Build history of the part. All positions in model axes, mm. A direction names the side the tool comes from. Round coordinates to 2 decimals unless told otherwise and drop trailing zeros. Loops run counter-clockwise (first coordinate to the right, second up) from the corner with the lowest first, then second, coordinate; pieces in that order, holes last. Notation, with made-up numbers: M 53,64.25 L 100,64.25 A20 cw 100,81.25 Z; hole C 8,71.25 d10. An arc over 180 degrees is marked long. Use one line per item in the form item = value. Start each with the question number.
Autodesk Inventor part; units mm, degrees
ref_plane "YZ Plane" through (0, 0, 0) normal (1, 0, 0) x (0, 1, 0)
ref_plane "XZ Plane" through (0, 0, 0) normal (0, 1, 0) x (-1, 0, 0)
ref_plane "XY Plane" through (0, 0, 0) normal (0, 0, 1) x (1, 0, 0)
sketch "Sketch1" plane through (0, 0, 0) normal (0, 0, 1) x (1, 0, 0)
  circle A0 centre (0, 0) radius 7.5
  line L0 (-10, 10) -> (10, 10)
  line L1 (10, 10) -> (10, -10)
  line L2 (10, -10) -> (-10, -10)
  line L3 (-10, -10) -> (-10, 10)
  line L4 (-10, -10) -> (-14, -10)
  line L5 (-14, -10) -> (-14, 10)
  line L6 (-14, 10) -> (-10, 10)
  line L7 (-10, 10) -> (-10, -10)
  line L8 (10, -10) -> (14, -10)
  line L9 (14, -10) -> (14, 10)
  line L10 (14, 10) -> (10, 10)
  line L11 (10, 10) -> (10, -10)
  line L12 (14, 10) -> (-14, 10)
  line L13 (-14, 10) -> (-14, 14)
  line L14 (-14, 14) -> (14, 14)
  line L15 (14, 14) -> (14, 10)
  line L16 (14, -10) -> (-14, -10)
  line L17 (-14, -10) -> (-14, -14)
  line L18 (-14, -14) -> (14, -14)
  line L19 (14, -14) -> (14, -10)
  dimension "d0" = 15
  dimension "d1" = 20
  dimension "d2" = 20
  dimension "d3" = 4
  dimension "d4" = 4
  dimension "d5" = 4
  dimension "d9" = 4
extrude "Extrusion1" add sketch "Sketch1" along normal blind 1
sketch "Sketch2" plane through (0, 0, 1) normal (0, 0, 1) x (1, 0, 0)
  circle A0 centre (0, 0) radius 7.5
  circle A1 centre (0, 0) radius 11
  line L0 (14, 14) -> (-14, 14)
  circle A2 centre (0, 0) radius 7.5
  line L1 (-14, 14) -> (-14, -14)
  line L2 (-14, -14) -> (14, -14)
  line L3 (14, -14) -> (14, 14)
  dimension "d8" = 22
extrude "Extrusion2" add sketch "Sketch2" along normal blind 7 contours L3 L2 L1 L0
sketch "Sketch3" plane through (0, 0, 0) normal (0, 0, -1) x (-1, 0, 0)
  line L0 (14, 14) -> (14, -14)
  line L1 (-14, 14) -> (14, 14)
  line L2 (-14, -14) -> (-14, 14)
  line L3 (14, -14) -> (-14, -14)
  circle A0 centre (0, 0) radius 7.5
  line L4 (10, 10) -> (10, -10)
  line L5 (10, -10) -> (-10, -10)
  line L6 (-10, -10) -> (-10, 10)
  line L7 (-10, 10) -> (10, 10)
  line L8 (-10, -10) -> (-10, -14)
  line L9 (10, -10) -> (10, -14)
  line L10 (14, -14) -> (-14, -14)
  dimension "d12" = 4
extrude "Extrusion3" add sketch "Sketch3" along normal blind 12 contours L0 L3 L9 L4 L7 L6 L8 L2 L1
fillet "Fillet1" radius 6 2 edges at (-12, -14, -12) (12, -14, -12)
fillet "Fillet2" radius 4 5 edges at (-14, 14, -2) (0, 14, 8) (14, 14, -2) (-14, 0, 8) (14, 0, 8)
sketch "Sketch4" plane through (-10, 10, 0) normal (0, -1, 0) x (1, 0, 0)
  line L0 (15, -3) -> (5, -3)
  line L1 (5, -3) -> (5, -9)
  line L2 (5, -9) -> (15, -9)
  line L3 (15, -9) -> (15, -3)
  line L4 (0, 0) -> (20, 0)
  line L5 (20, -12) -> (20, -6)
  point P0 (10, 0)
  dimension "d17" = 10
  dimension "d18" = 6
  dimension "d19" = 3
  dimension "d20" = 5
extrude "Extrusion4" cut sketch "Sketch4" against normal blind 10
fillet "Fillet3" radius 2 4 edges at (0, 14, -9) (-5, 14, -6) (5, 14, -6) (0, 14, -3)
properties part number "mocowanie lozyska 10-2"
Q1. Saw through at D-D (z = 2.25). Give the cut face in (x, y), and give its area (3 significant figures).
Q2. Tool access for faces 1 (the face through (-5.8, 13.6, -5.9)), 2 (the face through (-2.38, 10.74, 4.45)), 3 (the face through (-10, -2, -6)): list every direction of +Z, -Z, +X, -X, +Y, -Y with a clear straight run to the whole face (end or side of a thin tool).
Q3. Saw through at A-A (y = 0). Give the cut face in (x, z).
Q4. Drop flat-ended pins along their axis: P1, Ø12, axis at x = 9, z = -2, coming from the -Y side; P2, Ø9.5, axis at x = -0.5, z = -8, coming from the -Y side; P3, Ø5, axis at x = -5, y = 7, coming from the -Z side; P4, Ø2, axis at x = 0.5, y = 11, coming from the +Z side. Give the stop position or say it passes through.
Q5. Saw through at C-C (z = -6.5). Give the cut face in (x, y), and give its area (3 significant figures).
Q6. Pull direction Z, two halves, no side cores. Call faces 4 (the face through (0, 11, -9)), 5 (the face through (10, -2, -6)), 6 (the face through (-5, 11, -6)), 7 (the face through (7.2, 2.6, 1)): pulls with the +Z half, pulls with the -Z half, needs draft (parallel to the pull), parting line crosses it, or undercut.
Q7. Saw through at B-B (x = 0). Give the cut face in (y, z).
Q8. Wall check: probe 1 along Y at (x, z) = (0, 3.25); probe 2 along Y at (x, z) = (0, 0.6); probe 3 along X at (y, z) = (0.75, -5.5). Give the ranges that are in metal, low to high.
Filled in:
q1.outline = M -14,-14 L 14,-14 L 14,10 A4 ccw 10,14 L -10,14 A4 ccw -14,10 Z; hole C 0,0 d22
q1.area = 397 mm²
q2.face_1 = +Y
q2.face_2 = +Z
q2.face_3 = -Z, -Y
q3.outline = M -14,-12 L -10,-12 L -10,0 L -7.5,0 L -7.5,1 L -11,1 L -11,7.87 A4 ccw -14,4 Z; M 7.5,0 L 10,0 L 10,-12 L 14,-12 L 14,4 A4 ccw 11,7.87 L 11,1 L 7.5,1 Z
q4.P1 = -14
q4.P2 = 10
q4.P3 = 0
q4.P4 = 7.9
q5.outline = M -14,-13.98 L -10,-13.98 L -10,10 L -5,10 L -5,12 A2 ccw -7,14 L -10,14 A4 ccw -14,10 Z; M 5,10 L 10,10 L 10,-13.98 L 14,-13.98 L 14,10 A4 ccw 10,14 L 7,14 A2 ccw 5,12 Z
q5.area = 255 mm²
q6.face_4 = undercut
q6.face_5 = needs draft
q6.face_6 = undercut
q6.face_7 = pulls with the +Z half
q7.outline = M -14,0 L -7.5,0 L -7.5,1 L -11,1 L -11,8 L -14,8 Z; M 7.5,0 L 10,0 L 10,-3 L 12,-3 A2 ccw 14,-1 L 14,4 A4 ccw 11,7.87 L 11,1 L 7.5,1 Z; M 10,-12 L 14,-12 L 14,-11 A2 ccw 12,-9 L 10,-9 Z
q8.probe_1 = -14 to -11, 11 to 14
q8.probe_2 = -14 to -7.5, 7.5 to 14
q8.probe_3 = -14 to -10, 10 to 14
